```python
from build123d import *

# Parameters (mm, degrees)
SKETCH_1_R          = 1.7
EXTRUDE_1_DEPTH     = 7
SKETCH_2_R          = 14
EXTRUDE_2_DEPTH     = 5
CUT_EXTRUDE_1_REACH = 29.505
SKETCH_3_R          = 4
SKETCH_4_R          = 3.25
CUT_EXTRUDE_2_DEPTH = 4
CHAMFER_1_SIZE      = 1


with BuildPart() as part:
    # 草图1 → 凸台-拉伸1 (new body)
    with BuildSketch(Plane(origin=(0, 0, 0), x_dir=(1, 0, 0), z_dir=(0, 1, 0))):
        Polygon((0, 17.5), (12.905591591, 17.5), (17.5, 12.905591591), (17.5, 0), (17.5, -12.905591591), (12.905591591, -17.5), (0, -17.5), (-12.905591591, -17.5), (-17.5, -12.905591591), (-17.5, 0), (-17.5, 12.905591591), (-12.905591591, 17.5), align=None)
        with Locations(Location((12.426918465, 12.374368671, 0), (0, 0, 270))):
            Circle(SKETCH_1_R, mode=Mode.SUBTRACT)
        with Locations(Location((12.374368671, -12.426918465, 0), (0, 0, 270))):
            Circle(SKETCH_1_R, mode=Mode.SUBTRACT)
        with Locations(Location((-12.426918465, -12.374368671, 0), (0, 0, 270))):
            Circle(SKETCH_1_R, mode=Mode.SUBTRACT)
        with Locations(Location((-12.374368671, 12.426918465, 0), (0, 0, 270))):
            Circle(SKETCH_1_R, mode=Mode.SUBTRACT)
    extrude(amount=EXTRUDE_1_DEPTH)

    # 草图2 → 凸台-拉伸2 (add)
    with BuildSketch(Plane(origin=(0, 7, 0), x_dir=(1, 0, 0), z_dir=(0, 1, 0))):
        with Locations(Location((0, 0, 0), (0, 0, 270))):
            Circle(SKETCH_2_R)
    extrude(amount=EXTRUDE_2_DEPTH)

    # 草图3 → 切除-拉伸1 (cut, up to next)
    with BuildSketch(Plane(origin=(0, 12, 0), x_dir=(1, 0, 0), z_dir=(0, 1, 0)), mode=Mode.PRIVATE) as cut_extrude_1_sk1:
        with Locations(Location((0, 0, 0), (0, 0, 270))):
            Circle(SKETCH_3_R)
    cut_extrude_1_tool1 = extrude(cut_extrude_1_sk1.sketch, amount=-CUT_EXTRUDE_1_REACH, mode=Mode.PRIVATE) & part.part
    add(cut_extrude_1_tool1.solids().sort_by_distance((0, 12, 0))[0], mode=Mode.SUBTRACT)

    # 草图4 → 切除-拉伸2 (cut)
    with BuildSketch(Plane.XZ):
        with Locations(Location((-12.426918465, 12.374368671, 0), (0, 0, 270))):
            Circle(SKETCH_4_R)
        with Locations(Location((12.374368671, 12.426918465, 0), (0, 0, 270))):
            Circle(SKETCH_4_R)
        with Locations(Location((12.426918465, -12.374368671, 0), (0, 0, 270))):
            Circle(SKETCH_4_R)
        with Locations(Location((-12.374368671, -12.426918465, 0), (0, 0, 270))):
            Circle(SKETCH_4_R)
    extrude(amount=-CUT_EXTRUDE_2_DEPTH, mode=Mode.SUBTRACT)

    # 倒角1
    chamfer_1_edges = [part.edges().sort_by_distance(p)[0] for p in [
        (0, 12, -14),
    ]]
    chamfer(chamfer_1_edges, length=CHAMFER_1_SIZE)


solid = part.part
```
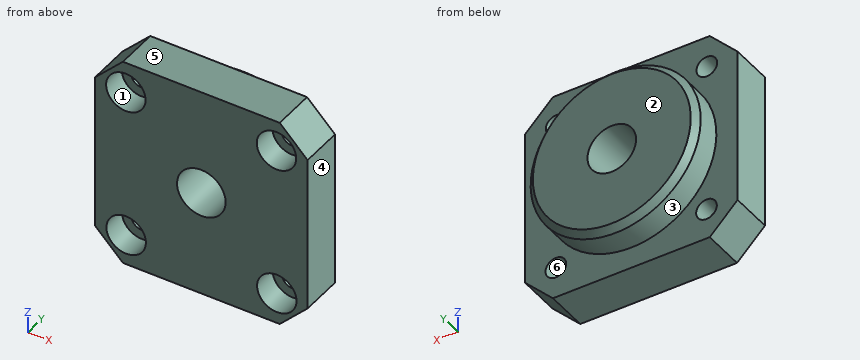
Geometry: final body of the model. Coordinates: model frame, mm. Face numbers are marked on the shaded views. A direction names the side the tool comes from. Round coordinates to 2 decimals unless told otherwise and drop trailing zeros. Write each loop counter-clockwise with the first axis right and the second up, starting at its lowest first coordinate (ties: lowest second). Pieces come first, ordered by that corner, then holes. Notation, with made-up numbers: (20, 48.25) -> (71, 48.25) arc R14 ccw to (71, 52.25) -> close; hole circle Ø3 at (38, 17.5). An arc over 180 degrees is marked (long way). Return JSON: item names as keys, results as strings.
Q1. Section A-A on z = 0. Return the cut outline in (x, y).
From the geometry:
{"outline": "(-17.5, 0) -> (-4, 0) -> (-4, 12) -> (-13, 12) -> (-14, 11) -> (-14, 7) -> (-17.5, 7) -> close; (4, 0) -> (17.5, 0) -> (17.5, 7) -> (14, 7) -> (14, 11) -> (13, 12) -> (4, 12) -> close"}
Q2. Set-up query: the marked faces 1, 2 and 3. Return all of +Z, -Z, +X, -X, +Y, -Y with unobstructed straight access to the full face (end or side cutting, diameter ignored); none if empty.
From the geometry:
{"face 1": "-Y", "face 2": "+Z, -Z, +X, -X, +Y", "face 3": "+Y"}
Q3. Section D-D on y = 9.25. Return the cut outline in (x, z), and give its area (3 significant figures).
From the geometry:
{"outline": "circle Ø28 at (0, 0); hole circle Ø8 at (0, 0)", "area": "565 mm2"}
Q4. Mould query, pull axis Z, two halves, no side actions, for the marked faces 4, 5 and 6. Classes: +Z half, -Z half, draft (parallel to the pull), parting line (faces both ways), or undercut.
From the geometry:
{"face 4": "draft", "face 5": "+Z half", "face 6": "undercut"}
Q5. Ray query, line 1 (X direction, y = 4.25, z = 13.5); line 2 (Z direction, x = -14, y = 2); line 3 (Z direction, x = 13.5, y = 3.25). Return the intervals inside material, ascending.
From the geometry:
{"line 1": "-16.91 to -13.7, -11.15 to 11.06, 13.69 to 16.91", "line 2": "-16.41 to -15.24, -9.61 to 9.53, 15.22 to 16.41", "line 3": "-16.91 to -15.44, -9.31 to 9.38, 15.48 to 16.91"}
Q6. Section C-C on y = 5. Return the cut outline in (x, z).
From the geometry:
{"outline": "(-17.5, -12.91) -> (-12.91, -17.5) -> (12.91, -17.5) -> (17.5, -12.91) -> (17.5, 12.91) -> (12.91, 17.5) -> (-12.91, 17.5) -> (-17.5, 12.91) -> close; hole circle Ø3.4 at (-12.43, 12.37); hole circle Ø3.4 at (-12.37, -12.43); hole circle Ø8 at (0, 0); hole circle Ø3.4 at (12.37, 12.43); hole circle Ø3.4 at (12.43, -12.37)"}
Q7. First-contact query: pin 1 Ø3 at (x, z) = (-12.5, 11.5) entering from -Y; pin 2 Ø2 at (y, z) = (2.5, -14) entering from +X; pin 3 Ø6 at (x, z) = (12.43, -12.37) entering from +Y; pin 4 Ø2.5 at (x, z) = (12.37, 12.43) entering from +Y. Flat tips, straight axial feed; report the tip coordinate or a pass-through.
From the geometry:
{"pin 1": "y = 4", "pin 2": "x = 17.41", "pin 3": "y = 7", "pin 4": "through"}
Q8. Section B-B on x = 0. Return the cut outline in (y, z).
From the geometry:
{"outline": "(0, -17.5) -> (7, -17.5) -> (7, -14) -> (11, -14) -> (12, -13) -> (12, -4) -> (0, -4) -> close; (0, 4) -> (12, 4) -> (12, 13) -> (11, 14) -> (7, 14) -> (7, 17.5) -> (0, 17.5) -> close"}
